Check sheet for the modelled part. Datum: model origin and axes. Units: mm. Face numbers are marked on the shaded views. Give positions to 0.01 mm unless a question says otherwise; leave off trailing zeros. Loops run counter-clockwise (first coordinate to the right, second up) from the corner with the lowest first, then second, coordinate; pieces in that order, holes last. Notation, with made-up numbers: M 65,85 L 115,85 A28 cw 115,113 Z; hole C -17,40 d2. An arc over 180 degrees is marked long. Use one line per item in the form item = value.
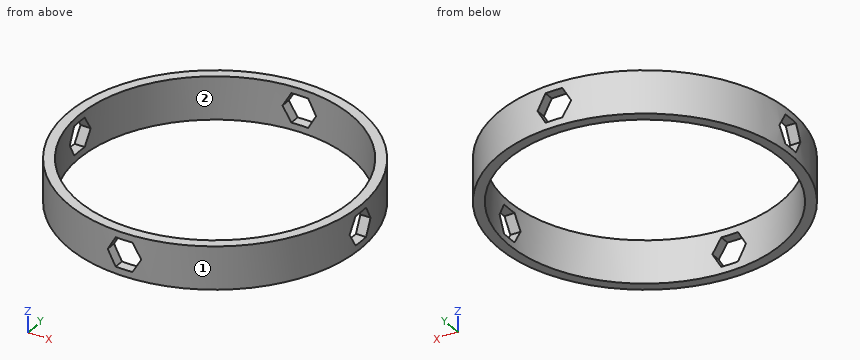
from build123d import *

# Parameters (mm, degrees)
SKETCH1_R           = 34.11
SKETCH1_R_2         = 31.75
BOSS_EXTRUDE1_DEPTH = 11.5
CUT_EXTRUDE1_DEPTH  = 10
CIRPATTERN2_COUNT   = 4
CUT_EXTRUDE2_START  = -1.5
SKETCH3_R           = 34.11
CUT_EXTRUDE2_DEPTH  = 1.5


with BuildPart() as part:
    # Sketch1 → Boss-Extrude1 (new body)
    with BuildSketch(Plane.XY):
        Circle(SKETCH1_R)
        Circle(SKETCH1_R_2, mode=Mode.SUBTRACT)
    extrude(amount=BOSS_EXTRUDE1_DEPTH)

    # Sketch2 → Cut-Extrude1 (cut)
    with BuildSketch(Plane(origin=(0, 34.11, 0), x_dir=(1, 0, 0), z_dir=(0, 1, 0))):
        Polygon((3.92598183, -5), (1.962990915, -1.6), (-1.962990915, -1.6), (-3.92598183, -5), (-1.962990915, -8.4), (1.962990915, -8.4), align=None)
    cut_extrude1 = extrude(amount=-CUT_EXTRUDE1_DEPTH, mode=Mode.SUBTRACT)

    # CirPattern2: Cut-Extrude1 ×4 about axis
    cirpattern2_axis = Axis((0, 0, 0), (0, 0, 1))
    for i in range(1, CIRPATTERN2_COUNT):
        add(cut_extrude1.rotate(cirpattern2_axis, i * 360 / CIRPATTERN2_COUNT), mode=Mode.SUBTRACT)

    # Sketch3 → Cut-Extrude2 (cut)
    with BuildSketch(Plane.XY.offset(11.5).offset(CUT_EXTRUDE2_START)):
        Circle(SKETCH3_R)
    extrude(amount=CUT_EXTRUDE2_DEPTH, mode=Mode.SUBTRACT)


solid = part.part
1) Scan lines: line 1 (Y direction, x = -24.5, z = 4.5); line 2 (X direction, y = -29, z = 3.75); line 3 (X direction, y = 22.5, z = 5.75). Record each from-to range of solid material in increasing order.
Evaluation:
line_1 = -23.73 to -20.19, 20.19 to 23.73
line_2 = -17.96 to -12.93, 12.93 to 17.96
line_3 = -25.64 to -22.4, 22.4 to 25.64
2) Section check C-C (y = 9). Record the cut outline in (x, z), then the cut area to 3 significant figures.
Evaluation:
outline = M -32.9,0 L -30.45,0 L -30.45,10 L -32.9,10 Z; M 30.45,0 L 32.9,0 L 32.9,10 L 30.45,10 Z
area = 49.1 mm^2
3) Release check for a two-part mould opening along Y. For the marked faces 1 and 2 record: pulls with the +Y half, pulls with the -Y half, needs draft (parallel to the pull), parting line crosses it, or undercut.
Evaluation:
face_1 = parting line crosses it
face_2 = undercut
4) Depth check by flat-ended pin: pin 1 Ø4 at (x, z) = (-24, 8.5) entering from +Y; pin 2 Ø6 at (x, z) = (-14.5, 4) entering from -Y; pin 3 Ø3 at (x, y) = (25.5, -26.5) entering from +Z; pin 4 Ø6 at (y, z) = (-21, 2.5) entering from -X. Enter the tip coordinate at first touch or a pass-through.
Evaluation:
pin_1 = 26.07
pin_2 = -32.11
pin_3 = through
pin_4 = -28.97
5) Section check D-D (x = -25). Record the cut outline in (y, z).
Evaluation:
outline = M -23.21,0 L -19.57,0 L -19.57,10 L -23.21,10 Z; M 19.57,0 L 23.21,0 L 23.21,10 L 19.57,10 Z
6) Section check A-A (x = 0). Record the cut outline in (y, z), then the cut area to 3 significant figures.
Evaluation:
outline = M -34.11,0 L -31.75,0 L -31.75,1.6 L -34.11,1.6 Z; M -34.11,8.4 L -31.75,8.4 L -31.75,10 L -34.11,10 Z; M 31.75,0 L 34.11,0 L 34.11,1.6 L 31.75,1.6 Z; M 31.75,8.4 L 34.11,8.4 L 34.11,10 L 31.75,10 Z
area = 15.1 mm^2
